Here's how the part is built. I have some questions about the finished solid (model axes, mm). A direction names the side the tool comes from. Give positions to 0.01 mm unless a question says otherwise; leave off trailing zeros. Loops run counter-clockwise (first coordinate to the right, second up) from the corner with the lowest first, then second, coordinate; pieces in that order, holes last. Notation, with made-up numbers: (52.25, 46.25) -> (105.25, 46.25) arc R28 ccw to (105.25, 83.25) -> close; hole circle Ø1 at (30, 1.5). An arc over 180 degrees is marked (long way). Answer in a Markdown table with one row per item. Add a question column.
Item 1: If we section it at B-B (y = 11): Write out the boundary of the cut face in (x, z), then the cut area to 3 significant figures.
Item 2: If we section it at A-A (x = -6.5): Write out the boundary of the cut face in (y, z), then the cut area to 3 significant figures.
Item 3: Which directions (+Z, -Z, +X, -X, +Y, -Y) give clear straight access to the entire face, cutting with the end or side of a thin tool? Please do faces 4 (the face through (2, 8, -1)), 5 (the face through (0.968, 7.4, -0.5)).
Item 4: If I drill on line 1 (Y direction, x = 0, z = -0.25); line 2 (X direction, y = 8.5, z = -0.6); line 3 (Y direction, x = 19.5, z = -0.25), over which ranges is the centre line in solid material (lowest first)?
Item 5: We'd pull the mould along Y, two halves only. Please class faces 1 (the face through (0.4, 0, -0.5)), 2 (the face through (24.968, 10.6, -0.5)), 3 (the face through (-10.232, 7.4, -0.5)): released by +Y, released by -Y, zero draft, split by the parting line, or undercut.
Item 6: If we section it at C-C (z = -0.5): Write out the boundary of the cut face in (x, y), then the cut area to 3 significant figures.
Item 7: If we section it at D-D (x = -24): Write out the boundary of the cut face in (y, z).
```python
from build123d import *

# Parameters (mm, degrees)
F1_DEPTH = 1
F3_R     = 0.4045
F3_R_2   = 0.404712
F4_DEPTH = 1.5
F5_W     = 11.2
F5_H     = 11.2
F6_DEPTH = 1


with BuildPart() as f1:
    # F0 (on Top) → F1 (new body)
    with BuildSketch(Plane.XY):
        with BuildLine():
            ThreePointArc((-34.23158, 6.248362), (-32.755389, 2.177921), (-29.013159, 0))
            Line((-29.013159, 0), (19.749998, 0))
            ThreePointArc((19.749998, 0), (23.492228, 2.177921), (24.96842, 6.248362))
            Line((24.96842, 6.248362), (24.96842, 15))
            Line((24.96842, 15), (-34.23158, 15))
            Line((-34.23158, 15), (-34.23158, 6.248362))
        make_face()
    extrude(amount=-F1_DEPTH)

    # F3 (on face) → F4 (join)
    with BuildSketch(Plane.XZ):
        with Locations((-19.013159, -0.5)):
            Circle(F3_R)
        with Locations((-4.630594, -0.5)):
            Circle(F3_R_2)
        with Locations((9.749998, -0.5)):
            Circle(F3_R)
    extrude(amount=F4_DEPTH)

    # F5 (on face) → F6 (cut)
    with BuildSketch(Plane.XY):
        with Locations((-4.63158, 7.5)):
            Rectangle(F5_W, F5_H)
    extrude(amount=-F6_DEPTH, mode=Mode.SUBTRACT)


solid = f1.part
```
Recorded:
| question | item | result |
|---|---|---|
| 1 | outline | (-34.23, -1) -> (-10.23, -1) -> (-10.23, 0) -> (-34.23, 0) -> close; (0.97, -1) -> (24.97, -1) -> (24.97, 0) -> (0.97, 0) -> close |
| 1 | area | 48.0 mm^2 |
| 2 | outline | (0, -1) -> (1.9, -1) -> (1.9, 0) -> (0, 0) -> close; (13.1, -1) -> (15, -1) -> (15, 0) -> (13.1, 0) -> close |
| 2 | area | 3.80 mm^2 |
| 3 | face 4 | -Z, +X, -X, +Y, -Y |
| 3 | face 5 | +Z, -Z |
| 4 | line 1 | y = 0 to 1.9, 13.1 to 15 |
| 4 | line 2 | x = -34.23 to -10.23, 0.97 to 24.97 |
| 4 | line 3 | y = 0 to 15 |
| 5 | face 1 | released by -Y |
| 5 | face 2 | zero draft |
| 5 | face 3 | undercut |
| 6 | outline | (-34.23, 6.25) arc R6.35 ccw to (-29.01, 0) -> (-19.42, 0) -> (-19.42, -1.5) -> (-18.61, -1.5) -> (-18.61, 0) -> (-5.04, 0) -> (-5.04, -1.5) -> (-4.23, -1.5) -> (-4.23, 0) -> (9.35, 0) -> (9.35, -1.5) -> (10.15, -1.5) -> (10.15, 0) -> (19.75, 0) arc R6.35 ccw to (24.97, 6.25) -> (24.97, 15) -> (-34.23, 15) -> close; hole (-10.23, 1.9) -> (0.97, 1.9) -> (0.97, 13.1) -> (-10.23, 13.1) -> close |
| 6 | area | 750 mm^2 |
| 7 | outline | (0, -1) -> (15, -1) -> (15, 0) -> (0, 0) -> close |
